Part model, mm, in its own coordinate system. A direction names the side the tool comes from. Coordinates: 2 decimals unless noted, no trailing zeros. Loops run counter-clockwise (first coordinate to the right, second up) from the corner with the lowest first, then second, coordinate; pieces in that order, holes last. Notation, with made-up numbers: (56.5, -22) -> (96.5, -22) arc R26 cw to (96.5, -5) -> close; hole circle Ø11 at (60.25, 10.5). An arc over 180 degrees is marked (long way). Use one line per item in the form item = value. Start each with the question number.
(1) Pin check, flat tips, straight feed: P1, Ø18, axis at x = 46, z = 15.5, coming from the -Y side; P2, Ø9.5, axis at y = 14, z = -2, coming from the -X side; P3, Ø2, axis at x = 20, y = 14, coming from the -Z side; P4, Ø12, axis at x = 24.5, y = 27, coming from the +Z side. Stop position of each tip, or through.
(2) Band-saw the part on D-D on y = 40. Give the cut face in (x, z), then the cut area to 3 significant figures.
(3) Band-saw the part on C-C on x = 52. Give the cut face in (y, z).
(4) Band-saw the part on A-A on z = 0. Give the cut face in (x, y).
(5) Mould opens along X. For faces 4 (the flat face through (50, 37, 25.513)), 5 (the cylindrical face through (36.876, 18.832, -1.804)), 6 (the flat face through (8.882, 30.755, 16.434)), 7 (the flat face through (15, 9, 0)) say: +X half, -X half, draft (parallel to the pull), parting line (faces both ways), or undercut.
(6) 3-axis set-ups, long thin cutter, end or side, ignore diameter. For faces 1 (the flat face through (67, 3, 11)), 2 (the flat face through (7, 19, 2)), 3 (the flat face through (45, 31, 8)): which of +Z, -Z, +X, -X, +Y, -Y reach the whole face in a straight line?
(7) Band-saw the part on B-B on y = 6. Give the cut face in (x, z).
(8) Drill centre lines: L1, parallel to Z at x = 53, y = 5.5; L2, parallel to Y at x = 46, z = 10.5; L3, parallel to Y at x = 9, z = -5. Where is each one in solid material? Low to high. Write a range as [from, to].
```python
from build123d import *

# Parameters (mm, degrees)
F0_R      = 7
F1_DEPTH  = 43
F2_W      = 81
F2_H      = 19
F3_DEPTH  = 19
F4_W      = 29
F4_H      = 37.6470717937
F5_DEPTH  = 19
F6_R      = 5.5
F7_DEPTH  = 43.001
F10_DEPTH = 12


with BuildPart() as f1:
    # F0 (on Front) → F1 (new body)
    with BuildSketch(Plane.XZ):
        with BuildLine():
            Line((17.5183015976, 14.9110507722), (0, 18))
            Line((0, 18), (-7, 18))
            Line((-7, 18), (-14, 11))
            Line((-14, 11), (-14, -7))
            Line((-14, -7), (-7, -14))
            Line((-7, -14), (20.5039936013, -14))
            ThreePointArc((20.5039936013, -14), (23.7692293823, -15.2134137678), (25.4496323427, -18.2647058824))
            ThreePointArc((25.4496323427, -18.2647058824), (27.3946303601, -25.2244414792), (31, -31.4872081702))
            Line((31, -31.4872081702), (38, -31.4872081702))
            Line((38, -31.4872081702), (67, 1.5127918298))
            Line((67, 1.5127918298), (67, 20.5127918298))
            Line((67, 20.5127918298), (62, 25.5127918298))
            Line((62, 25.5127918298), (38, 25.5127918298))
            ThreePointArc((38, 25.5127918298), (29.5516950708, 16.748872076), (17.5183015976, 14.9110507722))
        make_face()
        Circle(F0_R, mode=Mode.SUBTRACT)
    extrude(amount=-F1_DEPTH)

    # F2 (on face) → F3 (cut)
    with BuildSketch(Plane.XZ):
        with Locations((26.5, -23.5)):
            Rectangle(F2_W, F2_H)
    extrude(amount=-F3_DEPTH, mode=Mode.SUBTRACT)

    # F4 (on face) → F5 (cut)
    with BuildSketch(Plane.XZ):
        with Locations((0.5, 4.8235358968)):
            Rectangle(F4_W, F4_H)
    extrude(amount=-F5_DEPTH, mode=Mode.SUBTRACT)

    # F6 (on face) → F7 (cut, through all)
    with BuildSketch(Plane.XZ):
        with Locations((53, 11.5127918298)):
            Circle(F6_R)
    extrude(amount=-F7_DEPTH, mode=Mode.SUBTRACT)

    # F9 (on offset) → F10 (cut, symmetric)
    with BuildSketch(Plane.XZ.offset(-19)):
        with BuildLine():
            ThreePointArc((21.6885041445, 25.6739929318), (36.8569687391, -1.7884864667), (67, -10.4872081702))
            Line((67, -10.4872081702), (67, 25.5127918298))
            Line((67, 25.5127918298), (21.6885041445, 25.6739929318))
        make_face()
    extrude(amount=F10_DEPTH, both=True, mode=Mode.SUBTRACT)


solid = f1.part
```
A:
q1.P1 = 0
q1.P2 = 15
q1.P3 = -14
q1.P4 = 16.46
q2.outline = (-14, -7) -> (-7, -14) -> (20.5, -14) arc R5 cw to (25.45, -18.26) arc R29 ccw to (31, -31.49) -> (38, -31.49) -> (67, 1.51) -> (67, 20.51) -> (62, 25.51) -> (38, 25.51) arc R19 cw to (17.52, 14.91) -> (0, 18) -> (-7, 18) -> (-14, 11) -> close; hole circle Ø14 at (0, 0); hole circle Ø11 at (53, 11.51)
q2.area = 2,680 mm²
q3.outline = (0, -14) -> (19, -14) -> (19, -15.56) -> (43, -15.56) -> (43, 6.1) -> (31, 6.1) -> (31, -9.39) -> (7, -9.39) -> (7, 6.1) -> (0, 6.1) -> close; (0, 16.92) -> (7, 16.92) -> (7, 25.51) -> (0, 25.51) -> close; (31, 16.92) -> (43, 16.92) -> (43, 25.51) -> (31, 25.51) -> close
q4.outline = (-14, 19) -> (-7, 19) -> (-7, 43) -> (-14, 43) -> close; (7, 19) -> (15, 19) -> (15, 0) -> (65.67, 0) -> (65.67, 7) -> (34.76, 7) -> (34.76, 31) -> (65.67, 31) -> (65.67, 43) -> (7, 43) -> close
q5.face_4 = draft
q5.face_5 = +X half
q5.face_6 = undercut
q5.face_7 = -X half
q6.face_1 = +Z, -Z, +X, +Y, -Y
q6.face_2 = +Z, -Z, -X, -Y
q6.face_3 = +Z, +X
q7.outline = (15, -14) -> (53.37, -14) -> (67, 1.51) -> (67, 20.51) -> (62, 25.51) -> (38, 25.51) arc R19 cw to (17.52, 14.91) -> (15, 15.36) -> close; hole circle Ø11 at (53, 11.51)
q8.L1 = [-14, 6.01], [17.01, 25.51]
q8.L2 = [0, 7], [31, 43]
q8.L3 = [19, 43]
